Build history of the part. All positions in model axes, mm. A direction names the side the tool comes from. Give positions to 0.01 mm unless a question says otherwise; leave off trailing zeros. Order: outer loops, then holes, each group sorted by start corner. A loop starts at its lowest first (then second) coordinate and runs counter-clockwise, first axis right, second up. Notation, with made-up numbers: M -36.75,2.25 L 1.25,2.25 A33 cw 1.25,40.25 Z; hole C 54.5,73.25 d2. An arc over 180 degrees is marked long. Answer as CSV lines item,"result".
from build123d import *

# Parameters (mm, degrees)
SKETCH1_W                    = 65
SKETCH1_H                    = 120
BASE_FLANGE1_DEPTH           = 5
EDGE_FLANGE1_STRIP_W         = 30
EDGE_FLANGE1_STRIP_H         = 5
EDGE_FLANGE1_STRIP_CUT_DEPTH = 120
EDGE_FLANGE1_DEPTH           = 120
EDGE_FLANGE2_STRIP_W         = 30
EDGE_FLANGE2_STRIP_H         = 5
EDGE_FLANGE2_STRIP_CUT_DEPTH = 120
EDGE_FLANGE2_DEPTH           = 120


# Sheet-metal steps are written as plain solids
with BuildPart() as part:
    # Sketch1 → Base-Flange1 (new body)
    with BuildSketch(Plane.XY):
        with Locations((0, -60)):
            Rectangle(SKETCH1_W, SKETCH1_H)
    extrude(amount=-BASE_FLANGE1_DEPTH)

    # Edge-Flange1 strip (across the edge) → Edge-Flange1 strip cut (cut)
    with BuildSketch(Plane(origin=(32.5, -120, 0), x_dir=(-1, 0, 0), z_dir=(0, 1, 0))):
        with Locations((-10, -2.5)):
            Rectangle(EDGE_FLANGE1_STRIP_W, EDGE_FLANGE1_STRIP_H)
    extrude(amount=EDGE_FLANGE1_STRIP_CUT_DEPTH, mode=Mode.SUBTRACT)

    # Edge-Flange1 section (across the edge) → Edge-Flange1 (add)
    with BuildSketch(Plane(origin=(32.5, -120, 0), x_dir=(-1, 0, 0), z_dir=(0, 1, 0))):
        with BuildLine():
            Line((-5, 5), (-5, 25))
            Line((-5, 25), (0, 25))
            Line((0, 25), (0, 5))
            ThreePointArc((0, 5), (1.464466094, 1.464466094), (5, 0))
            Line((5, 0), (5, -5))
            ThreePointArc((5, -5), (-2.071067812, -2.071067812), (-5, 5))
        make_face()
    extrude(amount=EDGE_FLANGE1_DEPTH)

    # Edge-Flange2 strip (across the edge) → Edge-Flange2 strip cut (cut)
    with BuildSketch(Plane(origin=(-32.5, 0, 0), x_dir=(1, 0, 0), z_dir=(0, -1, 0))):
        with Locations((-10, -2.5)):
            Rectangle(EDGE_FLANGE2_STRIP_W, EDGE_FLANGE2_STRIP_H)
    extrude(amount=EDGE_FLANGE2_STRIP_CUT_DEPTH, mode=Mode.SUBTRACT)

    # Edge-Flange2 section (across the edge) → Edge-Flange2 (add)
    with BuildSketch(Plane(origin=(-32.5, 0, 0), x_dir=(1, 0, 0), z_dir=(0, -1, 0))):
        with BuildLine():
            Line((-5, 5), (-5, 25))
            Line((-5, 25), (0, 25))
            Line((0, 25), (0, 5))
            ThreePointArc((0, 5), (1.464466094, 1.464466094), (5, 0))
            Line((5, 0), (5, -5))
            ThreePointArc((5, -5), (-2.071067812, -2.071067812), (-5, 5))
        make_face()
    extrude(amount=EDGE_FLANGE2_DEPTH)


solid = part.part
Item 1: Probe line 1 along X through (y, z) = (-60, 9.25); line 2 along Z through (x, y) = (-23, -37); line 3 along X through (y, z) = (-53.5, 3.5). List the from-to ranges inside material, lowest first. Write a range as from..to.
Geometry says:
line 1,"x = -37.5..-32.5, 32.5..37.5"
line 2,"z = -5..0"
line 3,"x = -37.39..-32.27, 32.27..37.39"
Item 2: Band-saw the part on C-C (x = -13.5). Give the cut face in (y, z).
Geometry says:
outline,"M -120,-5 L 0,-5 L 0,0 L -120,0 Z"
Item 3: Band-saw the part on B-B (y = -21.5). Give the cut face in (x, z).
Geometry says:
outline,"M -37.5,5 A10 ccw -27.5,-5 L 27.5,-5 A10 ccw 37.5,5 L 37.5,25 L 32.5,25 L 32.5,5 A5 cw 27.5,0 L -27.5,0 A5 cw -32.5,5 L -32.5,25 L -37.5,25 Z"
Item 4: Pull direction X, two halves, no side cores. Call faces 3 (the flat face through (0, -120, -2)), 4 (the flat face through (0, -59, 0)), 5 (the flat face through (32.5, -61, 15)), 6 (the cylindrical face through (34.49, -60.84, -2.15)): released by +X, released by -X, zero draft, split by the parting line, or undercut.
Geometry says:
face 3,"zero draft"
face 4,"undercut"
face 5,"undercut"
face 6,"released by +X"
Item 5: Drop a flat-ended pin along its axis: pin 1 (1.5 mm diameter, centred on x = -29, y = -74.5, fed in from -Z). Give the stop position or say it passes through.
Geometry says:
pin 1,"stops at z = -4.97"
Item 6: Band-saw the part on A-A (z = 15.25). Give the cut face in (x, y).
Geometry says:
outline,"M -37.5,-120 L -32.5,-120 L -32.5,0 L -37.5,0 Z; M 32.5,-120 L 37.5,-120 L 37.5,0 L 32.5,0 Z"
Item 7: 3-axis set-ups, long thin cutter, end or side, ignore diameter. For faces 1 (the cylindrical face through (31.07, -60.84, 1.5)), 2 (the flat face through (35, -61, 25)): which of +Z, -Z, +X, -X, +Y, -Y reach the whole face in a straight line?
Geometry says:
face 1,"+Z, +Y, -Y"
face 2,"+Z, +X, -X, +Y, -Y"
